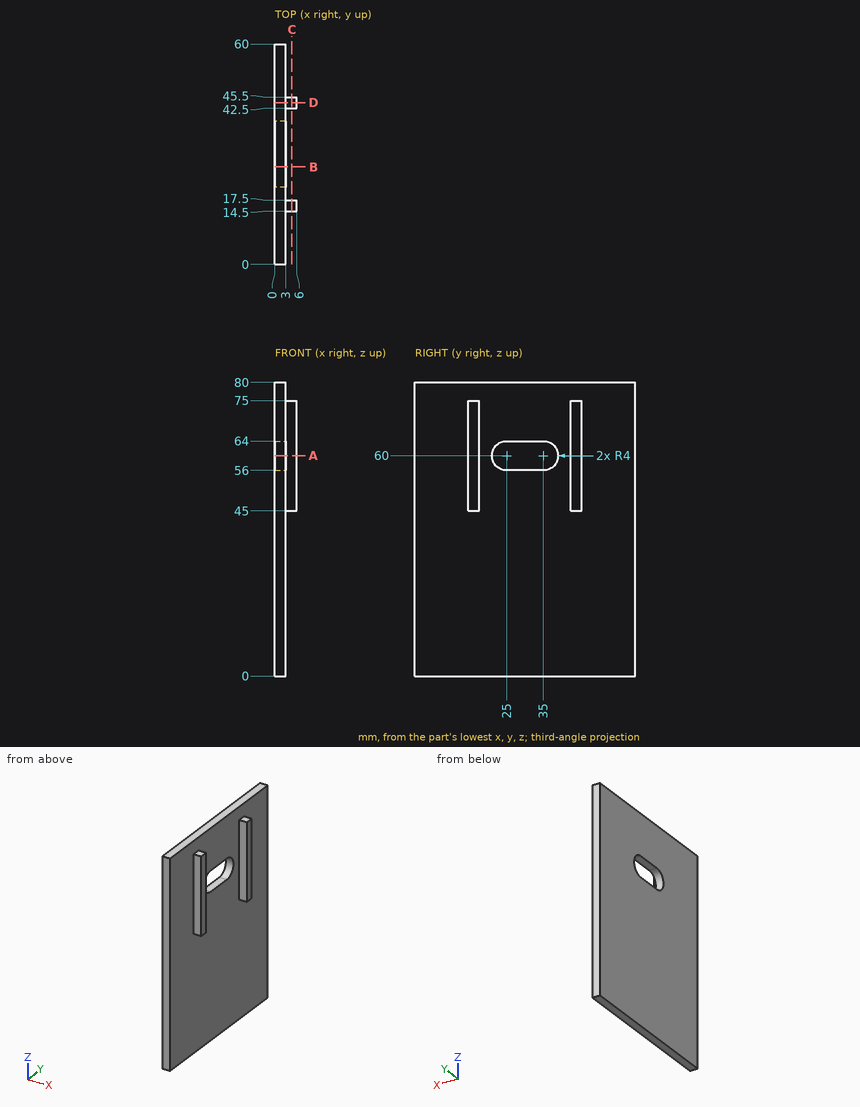
The drawing under review shows one solid part. Ordinate dimensions are in mm from its lowest x, y, z. Round coordinates to 2 decimals unless told otherwise and drop trailing zeros. Order: outer loops, then holes, each group sorted by start corner. A loop starts at its lowest first (then second) coordinate and runs counter-clockwise, first axis right, second up. Notation, with made-up numbers: (81, -11) -> (101, -11) arc R20 cw to (101, -1) -> close; hole circle Ø7 at (6.25, -39). An arc over 180 degrees is marked (long way). Return JSON: item names as keys, results as strings.
1. For L1, parallel to Y at x = 3.9, z = 49; L2, parallel to Z at x = 2.45, y = 26; L3, parallel to X at y = 45, z = 30, list the stretches that pass through material, from the lowest coordinate up. Write a range as [from, to].
Answer block:
{"L1": "y = [14.5, 17.5], [42.5, 45.5]", "L2": "z = [0, 56], [64, 80]", "L3": "x = [0, 3]"}
2. Take a section at A-A (z = 60). Write out the cut boundary in (x, y).
Answer block:
{"outline": "(0, 0) -> (3, 0) -> (3, 14.5) -> (6, 14.5) -> (6, 17.5) -> (3, 17.5) -> (3, 21) -> (0, 21) -> close; (0, 39) -> (3, 39) -> (3, 42.5) -> (6, 42.5) -> (6, 45.5) -> (3, 45.5) -> (3, 60) -> (0, 60) -> close"}
3. Take a section at D-D (y = 44). Write out the cut boundary in (x, z).
Answer block:
{"outline": "(0, 0) -> (3, 0) -> (3, 45) -> (6, 45) -> (6, 75) -> (3, 75) -> (3, 80) -> (0, 80) -> close"}
4. Take a section at B-B (y = 26.5). Write out the cut boundary in (x, z), then the cut area to 3 significant figures.
Answer block:
{"outline": "(0, 0) -> (3, 0) -> (3, 56) -> (0, 56) -> close; (0, 64) -> (3, 64) -> (3, 80) -> (0, 80) -> close", "area": "216 mm²"}
5. Take a section at C-C (x = 4.65). Write out the cut boundary in (y, z), then the cut area to 3 significant figures.
Answer block:
{"outline": "(14.5, 45) -> (17.5, 45) -> (17.5, 75) -> (14.5, 75) -> close; (42.5, 45) -> (45.5, 45) -> (45.5, 75) -> (42.5, 75) -> close", "area": "180 mm²"}
6. Insertion check: P1, Ø1.5, axis at x = 4, z = 66, coming from the -Y side; P2, Ø0.9, axis at x = 4.5, y = 44, coming from the +Z side; P3, Ø8, axis at y = 30.5, z = 36.5, coming from the +X side. Each pin has a flat end and moves straight along its axis. Give the tip position at first contact, or say it passes through.
Answer block:
{"P1": "stops at y = 14.5", "P2": "stops at z = 75", "P3": "stops at x = 3"}
